from build123d import *

# Parameters (mm, degrees)
MODEL_W             = 150
MODEL_H             = 120
MODEL_R             = 2
MODEL_R_2           = 1.5
BOSS_EXTRUDE1_DEPTH = 5
CUT_EXTRUDE1_DEPTH  = 216.636798312


with BuildPart() as part:
    # Model → Boss-Extrude1 (new body)
    with BuildSketch(Plane.XY):
        with Locations((90.051044639, 78.680861873)):
            Rectangle(MODEL_W, MODEL_H)
        with Locations((20.427424183, 93.680861873)):
            Circle(MODEL_R, mode=Mode.SUBTRACT)
        with Locations((26.427424183, 93.680861873)):
            Circle(MODEL_R, mode=Mode.SUBTRACT)
        with Locations((32.427424183, 93.680861873)):
            Circle(MODEL_R, mode=Mode.SUBTRACT)
        with Locations((20.427424183, 63.680861873)):
            Circle(MODEL_R, mode=Mode.SUBTRACT)
        with Locations((26.427424183, 63.680861873)):
            Circle(MODEL_R, mode=Mode.SUBTRACT)
        with Locations((32.427424183, 63.680861873)):
            Circle(MODEL_R, mode=Mode.SUBTRACT)
        with Locations((159.674665094, 93.680861873)):
            Circle(MODEL_R, mode=Mode.SUBTRACT)
        with Locations((153.674665094, 93.680861873)):
            Circle(MODEL_R, mode=Mode.SUBTRACT)
        with Locations((147.674665094, 93.680861873)):
            Circle(MODEL_R, mode=Mode.SUBTRACT)
        with Locations((159.674665094, 63.680861873)):
            Circle(MODEL_R, mode=Mode.SUBTRACT)
        with Locations((153.674665094, 63.680861873)):
            Circle(MODEL_R, mode=Mode.SUBTRACT)
        with Locations((147.674665094, 63.680861873)):
            Circle(MODEL_R, mode=Mode.SUBTRACT)
        with Locations((20.005670629, 133.907298569)):
            Circle(MODEL_R_2, mode=Mode.SUBTRACT)
        with Locations((160.096418648, 133.907298569)):
            Circle(MODEL_R_2, mode=Mode.SUBTRACT)
        with Locations((20.005670629, 23.454425177)):
            Circle(MODEL_R_2, mode=Mode.SUBTRACT)
        with Locations((160.096418648, 23.454425177)):
            Circle(MODEL_R_2, mode=Mode.SUBTRACT)
    extrude(amount=BOSS_EXTRUDE1_DEPTH)

    # Sketch3 → Cut-Extrude1 (cut, through all)
    with BuildSketch(Plane.XY.offset(5)):
        with BuildLine():
            Line((59.848510467, 125.37915187), (120.08763082, 125.37915187))
            ThreePointArc((120.08763082, 125.37915187), (122.560781495, 122.906001195), (120.08763082, 120.43285052))
            Line((120.08763082, 120.43285052), (59.848510467, 120.43285052))
            ThreePointArc((59.848510467, 120.43285052), (57.375359792, 122.906001195), (59.848510467, 125.37915187))
        make_face()
        with BuildLine():
            Line((59.848510467, 37.411582635), (120.08763082, 37.411582635))
            ThreePointArc((120.08763082, 37.411582635), (122.355268775, 35.14394468), (120.08763082, 32.876306725))
            Line((120.08763082, 32.876306725), (59.848510467, 32.876306725))
            ThreePointArc((59.848510467, 32.876306725), (57.580872512, 35.14394468), (59.848510467, 37.411582635))
        make_face()
    extrude(amount=-CUT_EXTRUDE1_DEPTH, mode=Mode.SUBTRACT)


solid = part.part
Verification items for the finished model (mm, model axes). A direction names the side the tool comes from. Round coordinates to 2 decimals unless told otherwise and drop trailing zeros. Write each loop counter-clockwise with the first axis right and the second up, starting at its lowest first coordinate (ties: lowest second). Pieces come first, ordered by that corner, then holes.
(1) Section check A-A (x = 111). Enter the section's corners in (y, z), plus the area to 3 significant figures.
Returned:
outline: (18.68, 0) - (32.88, 0) - (32.88, 5) - (18.68, 5) - close; (37.41, 0) - (120.43, 0) - (120.43, 5) - (37.41, 5) - close; (125.38, 0) - (138.68, 0) - (138.68, 5) - (125.38, 5) - close
area: 553 mm2
(2) Depth check by flat-ended pin: pin 1 Ø4.5 at (x, y) = (153.67, 63.68) entering from +Z; pin 2 Ø2.5 at (x, y) = (20.01, 23.45) entering from +Z. Enter the tip coordinate at first touch or a pass-through.
Returned:
pin 1: stops at z = 5
pin 2: passes through
(3) Material ranges on line 1 (Y direction, x = 75, z = 2.3); line 2 (X direction, y = 35.5, z = 4); line 3 (X direction, y = 133.5, z = 4.2), recorded low to high.
Returned:
line 1: y = 18.68 to 32.88, 37.41 to 120.43, 125.38 to 138.68
line 2: x = 15.05 to 57.61, 122.33 to 165.05
line 3: x = 15.05 to 18.56, 21.45 to 158.65, 161.54 to 165.05
(4) Access from +Z, -Z, +X, -X, +Y, -Y to the whole of each face (thin tool, end or side, straight path). Record for faces 1 (the flat face through (89, 80, 5)), 2 (the cylindrical face through (122.56, 122.96, 2.54)).
Returned:
face 1: +Z, +X, -X, +Y, -Y
face 2: +Z, -Z
(5) Mould release check, pull along Y, two halves, no side actions. Record for faces 3 (the flat face through (90, 32.876, 3)), 4 (the flat face through (89, 138.681, 2)), 5 (the flat face through (89, 18.681, 2)): pulls with the +Y half, pulls with the -Y half, needs draft (parallel to the pull), parting line crosses it, or undercut.
Returned:
face 3: undercut
face 4: pulls with the +Y half
face 5: pulls with the -Y half
(6) Section check B-B (y = 123). Enter the section's corners in (x, z).
Returned:
outline: (15.05, 0) - (57.38, 0) - (57.38, 5) - (15.05, 5) - close; (122.56, 0) - (165.05, 0) - (165.05, 5) - (122.56, 5) - close
(7) Section check C-C (z = 3.9). Give the number of separate pieces and of enclosed holes in the cut face, plus the area to 3 significant figures.
Returned:
separate pieces: 1
enclosed holes: 18
area: 17,200 mm2
